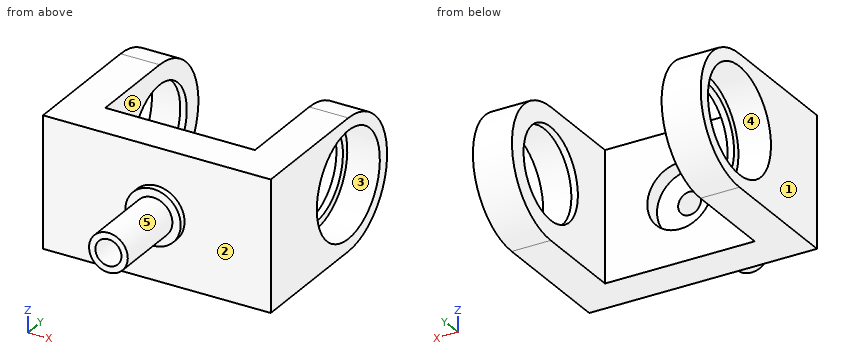
from build123d import *

# Parameters (mm, degrees)
SKETCH005_AS_DRAWN_R                 = 10
EXTRUDE005_DEPTH                     = 5
EXTRUDE005_ONTO_SKETCH005_ROLL_ANGLE = 90
SKETCH001_AS_DRAWN_W                 = 40
SKETCH001_AS_DRAWN_H                 = 70
SKETCH001_AS_DRAWN_R                 = 3.5
EXTRUDE002_DEPTH                     = 12
EXTRUDE002_ONTO_SKETCH001_ROLL_ANGLE = 90
SKETCH004_AS_DRAWN_R                 = 8.5
SKETCH004_AS_DRAWN_R_2               = 3.5
EXTRUDE004_DEPTH                     = 2
EXTRUDE004_ONTO_SKETCH004_ROLL_ANGLE = 90
SKETCH003_AS_DRAWN_R                 = 5.95
SKETCH003_AS_DRAWN_R_2               = 4
EXTRUDE003_DEPTH                     = 25
EXTRUDE003_ONTO_SKETCH003_ROLL_ANGLE = 90
CYLINDER001_R                        = 16.25
CYLINDER001_DEPTH                    = 10
SKETCH_R                             = 14
EXTRUDE_DEPTH                        = 12
CYLINDER_R                           = 16.25
CYLINDER_DEPTH                       = 10
EXTRUDE001_DEPTH                     = 12
FUSION_PITCH_ANGLE                   = 90


with BuildPart() as contra_nut_cut:
    # Sketch005 as drawn → Extrude005 (new)
    with BuildSketch(Plane.XY):
        Circle(SKETCH005_AS_DRAWN_R)
    extrude(amount=-EXTRUDE005_DEPTH)


with BuildPart() as contra_nut_cut_1:
    # Extrude005 onto Sketch005 roll: moved
    add(contra_nut_cut.part.rotate(Axis((0, 0, 0), (1, 0, 0)), EXTRUDE005_ONTO_SKETCH005_ROLL_ANGLE))


with BuildPart() as contra_nut_cut_2:
    # Extrude005 onto Sketch005 placement: moved
    add(contra_nut_cut_1.part)


with BuildPart() as contra_nut_cut_3:
    # Extrude005 placement: moved
    add(contra_nut_cut_2.part.moved(Location((0, -33, 0))))


with BuildPart() as nut_cut:
    # Sketch001 as drawn → Extrude002 (new)
    with BuildSketch(Plane.XY):
        Rectangle(SKETCH001_AS_DRAWN_W, SKETCH001_AS_DRAWN_H)
        Circle(SKETCH001_AS_DRAWN_R, mode=Mode.SUBTRACT)
    extrude(amount=-EXTRUDE002_DEPTH)


with BuildPart() as nut_cut_1:
    # Extrude002 onto Sketch001 roll: moved
    add(nut_cut.part.rotate(Axis((0, 0, 0), (1, 0, 0)), EXTRUDE002_ONTO_SKETCH001_ROLL_ANGLE))


with BuildPart() as nut_cut_2:
    # Extrude002 onto Sketch001 placement: moved
    add(nut_cut_1.part)


with BuildPart() as nut_cut_3:
    # Extrude002 placement: moved
    add(nut_cut_2.part.moved(Location((0, -40, 0))))

    # Cut002: cut contra-nut-cut
    add(contra_nut_cut_3.part, mode=Mode.SUBTRACT)


with BuildPart() as z_bearings_pad:
    # Sketch004 as drawn → Extrude004 (new)
    with BuildSketch(Plane.XY):
        Circle(SKETCH004_AS_DRAWN_R)
        Circle(SKETCH004_AS_DRAWN_R_2, mode=Mode.SUBTRACT)
    extrude(amount=-EXTRUDE004_DEPTH)


with BuildPart() as z_bearings_pad_1:
    # Extrude004 onto Sketch004 roll: moved
    add(z_bearings_pad.part.rotate(Axis((0, 0, 0), (1, 0, 0)), EXTRUDE004_ONTO_SKETCH004_ROLL_ANGLE))


with BuildPart() as z_bearings_pad_2:
    # Extrude004 onto Sketch004 placement: moved
    add(z_bearings_pad_1.part)


with BuildPart() as z_bearings_pad_3:
    # Extrude004 placement: moved
    add(z_bearings_pad_2.part.moved(Location((0, -42, 0))))


with BuildPart() as z_bearings_cylinder:
    # Sketch003 as drawn → Extrude003 (new)
    with BuildSketch(Plane.XY):
        Circle(SKETCH003_AS_DRAWN_R)
        Circle(SKETCH003_AS_DRAWN_R_2, mode=Mode.SUBTRACT)
    extrude(amount=-EXTRUDE003_DEPTH)


with BuildPart() as z_bearings_cylinder_1:
    # Extrude003 onto Sketch003 roll: moved
    add(z_bearings_cylinder.part.rotate(Axis((0, 0, 0), (1, 0, 0)), EXTRUDE003_ONTO_SKETCH003_ROLL_ANGLE))


with BuildPart() as z_bearings_cylinder_2:
    # Extrude003 onto Sketch003 placement: moved
    add(z_bearings_cylinder_1.part)


with BuildPart() as z_bearings_cylinder_3:
    # Extrude003 placement: moved
    add(z_bearings_cylinder_2.part.moved(Location((0, -65, 0))))


with BuildPart() as cylinder001:
    # Cylinder001 → Cylinder001 (new body)
    with BuildSketch(Plane.XY.offset(2)):
        Circle(CYLINDER001_R)
    extrude(amount=CYLINDER001_DEPTH)


with BuildPart() as bearing_nest_r_cut:
    # Sketch → Extrude (new body)
    with BuildSketch(Plane.XY):
        with BuildLine():
            ThreePointArc((20, 0), (0, 20), (-20, 0))
            Line((-20, 0), (-20, -40))
            Line((-20, -40), (20, -40))
            Line((20, -40), (20, 0))
        make_face()
        Circle(SKETCH_R, mode=Mode.SUBTRACT)
    extrude(amount=EXTRUDE_DEPTH)

    # Cut001: cut Cylinder001
    add(cylinder001.part, mode=Mode.SUBTRACT)


with BuildPart() as bearing_nest_r_cut_1:
    # Cut001 placement: moved
    add(bearing_nest_r_cut.part.moved(Location((0, 0, 23))))


with BuildPart() as cylinder:
    # Cylinder → Cylinder (new body)
    with BuildSketch(Plane.XY):
        Circle(CYLINDER_R)
    extrude(amount=CYLINDER_DEPTH)


with BuildPart() as fusion:
    # Sketch → Extrude001 (new body)
    with BuildSketch(Plane.XY):
        with BuildLine():
            ThreePointArc((20, 0), (0, 20), (-20, 0))
            Line((-20, 0), (-20, -40))
            Line((-20, -40), (20, -40))
            Line((20, -40), (20, 0))
        make_face()
        Circle(SKETCH_R, mode=Mode.SUBTRACT)
    extrude(amount=EXTRUDE001_DEPTH)

    # Cut: cut Cylinder
    add(cylinder.part, mode=Mode.SUBTRACT)


with BuildPart() as fusion_1:
    # Cut placement: moved
    add(fusion.part.moved(Location((0, 0, -35))))

    # Fusion: union nut-cut, z-bearings-pad, z-bearings-cylinder, bearing-nest-r-cut
    add(nut_cut_3.part)
    add(z_bearings_pad_3.part)
    add(z_bearings_cylinder_3.part)
    add(bearing_nest_r_cut_1.part)


with BuildPart() as fusion_2:
    # Fusion pitch: moved
    add(fusion_1.part.rotate(Axis((0, 0, 0), (0, 1, 0)), FUSION_PITCH_ANGLE))


with BuildPart() as fusion_3:
    # Fusion placement: moved
    add(fusion_2.part)


solid = fusion_3.part
Geometry: final body of the model. Coordinates: model frame, mm. Face numbers are marked on the shaded views. A direction names the side the tool comes from. Give positions to 0.01 mm unless a question says otherwise; leave off trailing zeros. Order: outer loops, then holes, each group sorted by start corner. A loop starts at its lowest first (then second) coordinate and runs counter-clockwise, first axis right, second up. Notation, with made-up numbers: (-13.5, 47.25) - (10.5, 47.25) arc R17 cw to (10.5, 73.25) - close; hole circle Ø6 at (47, 33). An arc over 180 degrees is marked (long way). Use CSV: the item, a comma, the result in double quotes.
1. Mould query, pull axis Y, two halves, no side actions, for the marked faces 1, 2 and 3. Classes: +Y half, -Y half, draft (parallel to the pull), parting line (faces both ways), or undercut.
Answers below:
face 1,"draft"
face 2,"-Y half"
face 3,"undercut"
2. Section query C-C (z = 12.5). Output: boundary loops of the cut face in (x, y).
Answers below:
outline,"(-35, -40) - (35, -40) - (35, -10.38) - (25, -10.38) - (25, -6.3) - (23, -6.3) - (23, -28) - (-23, -28) - (-23, -6.3) - (-25, -6.3) - (-25, -10.38) - (-35, -10.38) - close; (-35, 10.38) - (-25, 10.38) - (-25, 6.3) - (-23, 6.3) - (-23, 15.61) - (-35, 15.61) - close; (23, 6.3) - (25, 6.3) - (25, 10.38) - (35, 10.38) - (35, 15.61) - (23, 15.61) - close"
3. Contact query for flat-ended pins moving along their axis: pin 1 (10 mm diameter, centred on x = 18.5, y = -42.5, fed in from +Z); pin 2 (10 mm diameter, centred on y = -50, z = -3, fed in from -X); pin 3 (1 mm diameter, centred on x = 25.5, z = -12.5, fed in from -Y); pin 4 (6.5 mm diameter, centred on x = 0, z = 0, fed in from +Y). Output: stop coordinate, or through.
Answers below:
pin 1,"z = 20"
pin 2,"x = -5.95"
pin 3,"y = -40"
pin 4,"through"
4. Section query D-D (x = 30). Output: boundary loops of the cut face in (y, z).
Answers below:
outline,"(-40, -20) - (0, -20) arc R20 ccw to (0, 20) - (-40, 20) - close; hole circle Ø32.5 at (0, 0)"
5. Section query B-B (y = 2). Output: boundary loops of the cut face in (x, z).
Answers below:
outline,"(-35, -19.9) - (-23, -19.9) - (-23, -13.86) - (-25, -13.86) - (-25, -16.13) - (-35, -16.13) - close; (-35, 16.13) - (-25, 16.13) - (-25, 13.86) - (-23, 13.86) - (-23, 19.9) - (-35, 19.9) - close; (23, -19.9) - (35, -19.9) - (35, -16.13) - (25, -16.13) - (25, -13.86) - (23, -13.86) - close; (23, 13.86) - (25, 13.86) - (25, 16.13) - (35, 16.13) - (35, 19.9) - (23, 19.9) - close"
6. Section query A-A (x = 0). Output: boundary loops of the cut face in (y, z).
Answers below:
outline,"(-65, -5.95) - (-42, -5.95) - (-42, -8.5) - (-40, -8.5) - (-40, -20) - (-28, -20) - (-28, -10) - (-33, -10) - (-33, -3.5) - (-42, -3.5) - (-42, -4) - (-65, -4) - close; (-65, 4) - (-42, 4) - (-42, 3.5) - (-33, 3.5) - (-33, 10) - (-28, 10) - (-28, 20) - (-40, 20) - (-40, 8.5) - (-42, 8.5) - (-42, 5.95) - (-65, 5.95) - close"
7. Access query for the marked faces 4, 5 and 6. Directions: +Z, -Z, +X, -X, +Y, -Y. A direction counts if a zero-diameter tool reaches every point of the face in a straight line with its end or side. Return the directions, or none.
Answers below:
face 4,"-X"
face 5,"-Y"
face 6,"+Z, -Z, +Y"
8. Material intervals for line 1 along Y through (x, z) = (28, 0); line 2 along X through (y, z) = (-27.5, 3.5); line 3 along X through (y, z) = (-51, 0), sorted ascending. Write a range as from..to.
Answers below:
line 1,"-40..-16.25, 16.25..20"
line 2,"-35..-23, 23..35"
line 3,"-5.95..-4, 4..5.95"
